The listing builds one solid part. Answer for the finished solid, in the listing's coordinates (mm). A direction names the side the tool comes from. Coordinates: 2 decimals unless noted, no trailing zeros. Write each loop counter-clockwise with the first axis right and the second up, starting at its lowest first coordinate (ties: lowest second). Pieces come first, ordered by that corner, then holes. Notation, with made-up numbers: M 47,42 L 58,42 A12 ccw 58,54 Z; hole C 79,40 d4. An arc over 180 degrees is marked long. Write item = value, one per line. Start each with the question number.
```python
from build123d import *

# Parameters (mm, degrees)
F0_R      = 12.7
F1_DEPTH  = 76.2
F2_R      = 19.868023
F3_DEPTH  = 6.35
F4_R      = 19.76611
F5_DEPTH  = 6.35
F6_R      = 5.68078
F7_DEPTH  = 508
F7_FACE_R = 5.68078
F8_DEPTH  = 1270


with BuildPart() as f1:
    # F0 (on Top) → F1 (new body)
    with BuildSketch(Plane.XY):
        Circle(F0_R)
    extrude(amount=F1_DEPTH)

    # F2 (on Top) → F3 (join)
    with BuildSketch(Plane.XY):
        Circle(F2_R)
    extrude(amount=F3_DEPTH)

    # F4 (on face) → F5 (join)
    with BuildSketch(Plane.XY.offset(76.2)):
        Circle(F4_R)
    extrude(amount=F5_DEPTH)

    # F6 (on Front) → F7 (cut)
    with BuildSketch(Plane.XZ):
        with Locations((0, 41.454975)):
            Circle(F6_R)
    extrude(amount=-F7_DEPTH, mode=Mode.SUBTRACT)

    # F7_face (on face) → F8 (cut)
    with BuildSketch(Plane(origin=(0, 0, 41.454975), x_dir=(1, 0, 0), z_dir=(0, 1, 0))):
        Circle(F7_FACE_R)
    extrude(amount=-F8_DEPTH, mode=Mode.SUBTRACT)


solid = f1.part
```
1. The part is cut by section B-B, the plane y = 0. Write down the section's boundary in (x, z), and give its area (3 significant figures).
2. The part is cut by section C-C, the plane y = 15. Write down the section's boundary in (x, z), and give its area (3 significant figures).
3. The part is cut by section D-D, the plane x = -10. Write down the section's boundary in (y, z), and give its area (3 significant figures).
4. For faces 4 (the face through (5.42, -0.18, 43.16)), 5 (the face through (-15.686, -12.027, 79.331)), 6 (the face through (12.114, 3.815, 40.786)), determine the directions among +Z, -Z, +X, -X, +Y, -Y from which every point of the face is accessible in a straight line to the end or side of a thin tool.
5. Each of these flat-tipped pins is pushed along its axis until it touches: pin 1 (10 mm diameter, centred on y = -15, z = 69.5, fed in from -X); pin 2 (6 mm diameter, centred on y = 1, z = 55.5, fed in from +X); pin 3 (5 mm diameter, centred on y = -11, z = 60.5, fed in from +X). Where does it stop, or does it pass through?
6. For a pull along Z with two mould halves and no side action, classify faces 1 (the face through (-14.64, 13.43, 3.13)), 2 (the face through (0, 0, 82.55)), 3 (the face through (0, -13, 6.35)) as pulls with the +Z half, pulls with the -Z half, needs draft (parallel to the pull), parting line crosses it, or undercut.
7. Straight lines are drawn through the part: L1, parallel to Z at x = 6.5, y = -17; L2, parallel to Z at x = 0, y = -6.25; L3, parallel to X at y = -8, z = 39. For each, find the intervals that lie inside material, in ascending order. Write a range as [from, to].
8. The part is cut by section A-A, the plane x = 0. Write down the section's boundary in (y, z), and give its area (3 significant figures).
Solution:
q1.outline = M -19.87,0 L 19.87,0 L 19.87,6.35 L 12.7,6.35 L 12.7,76.2 L 19.77,76.2 L 19.77,82.55 L -19.77,82.55 L -19.77,76.2 L -12.7,76.2 L -12.7,6.35 L -19.87,6.35 Z; hole C 0,41.45 d11.36
q1.area = 2,180 mm^2
q2.outline = M -13.03,0 L 13.03,0 L 13.03,6.35 L -13.03,6.35 Z; M -12.87,76.2 L 12.87,76.2 L 12.87,82.55 L -12.87,82.55 Z
q2.area = 329 mm^2
q3.outline = M -17.17,0 L 17.17,0 L 17.17,6.35 L 7.83,6.35 L 7.83,76.2 L 17.05,76.2 L 17.05,82.55 L -17.05,82.55 L -17.05,76.2 L -7.83,76.2 L -7.83,6.35 L -17.17,6.35 Z
q3.area = 1,530 mm^2
q4.face_4 = +Y, -Y
q4.face_5 = +Z
q4.face_6 = none
q5.pin_1 = -7.83
q5.pin_2 = 12.7
q5.pin_3 = 9.44
q6.face_1 = needs draft
q6.face_2 = pulls with the +Z half
q6.face_3 = undercut
q7.L1 = [0, 6.35], [76.2, 82.55]
q7.L2 = [0, 35.77], [47.14, 82.55]
q7.L3 = [-9.86, -5.12], [5.12, 9.86]
q8.outline = M -19.87,0 L 19.87,0 L 19.87,6.35 L 12.7,6.35 L 12.7,35.77 L -12.7,35.77 L -12.7,6.35 L -19.87,6.35 Z; M -19.77,76.2 L -12.7,76.2 L -12.7,47.14 L 12.7,47.14 L 12.7,76.2 L 19.77,76.2 L 19.77,82.55 L -19.77,82.55 Z
q8.area = 1,990 mm^2
